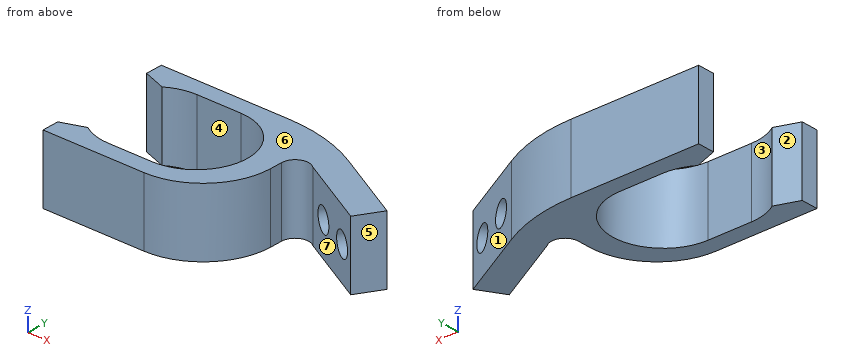
from build123d import *

# Parameters (mm, degrees)
F1_DEPTH = 5
F2_R     = 1.75
F3_DEPTH = 9.9
F4_R     = 24


# Not quite as in the source:
# - a feature names something its author has since deleted; it is built from what else it names


with BuildPart() as f1:
    # F0 (on Top) → F1 (new body, symmetric)
    with BuildSketch(Plane.XY):
        with BuildLine():
            Line((16.2096246684, 11.2512872423), (0, 20))
            Line((0, 20), (-25, 20))
            Line((-25, 20), (-25, 17.5))
            Line((-25, 17.5), (-17.5, 17.5))
            Line((-17.5, 17.5), (-11, 17.5))
            Line((-11, 17.5), (-3.5, 17.5))
            Line((-3.5, 17.5), (-3.5, 10))
            Line((-3.5, 10), (-3.5, 2.5))
            Line((-3.5, 2.5), (-11, 2.5))
            Line((-11, 2.5), (-17.5, 2.5))
            Line((-17.5, 2.5), (-25, 2.5))
            Line((-25, 2.5), (-25, 0))
            Line((-25, 0), (-10, 0))
            ThreePointArc((-10, 0), (-2.9289321881, 2.9289321881), (0, 10))
            Line((0, 10), (0, 11.8892861952))
            ThreePointArc((0, 11.8892861952), (1.1623016269, 13.7053978206), (3.2982614357, 13.4106399491))
            Line((3.2982614357, 13.4106399491), (14.0066361954, 7.6310801635))
            Line((14.0066361954, 7.6310801635), (16.2096246684, 11.2512872423))
        make_face()
        with BuildLine():
            Line((-17.5, 17.5), (-25, 17.5))
            Line((-25, 17.5), (-21.614659653, 16.270532349))
            ThreePointArc((-21.614659653, 16.270532349), (-19.6472083483, 17.186062643), (-17.5, 17.5))
        make_face()
        with BuildLine():
            Line((-21.614659653, 3.729467651), (-25, 2.5))
            Line((-25, 2.5), (-17.5, 2.5))
            ThreePointArc((-17.5, 2.5), (-19.6472083483, 2.813937357), (-21.614659653, 3.729467651))
        make_face()
        with BuildLine():
            Line((-3.5, 17.5), (-11, 17.5))
            ThreePointArc((-11, 17.5), (-5.6966991411, 15.3033008589), (-3.5, 10))
            Line((-3.5, 10), (-3.5, 17.5))
        make_face()
        with BuildLine():
            Line((-3.5, 2.5), (-3.5, 10))
            ThreePointArc((-3.5, 10), (-5.6966991411, 4.6966991411), (-11, 2.5))
            Line((-11, 2.5), (-3.5, 2.5))
        make_face()
    extrude(amount=F1_DEPTH, both=True)

    # F2 (on face) → F3 (cut)
    with BuildSketch(Plane(origin=(8.3593712251, 15.4882522465, 0), x_dir=(-0.8800071661, 0.4749604064, 0), z_dir=(0.4749604064, 0.8800071661, 0))):
        with Locations((-5.9206699059, 0)):
            Circle(F2_R)
        with Locations((0.0793300941, 0)):
            Circle(F2_R)
    extrude(amount=-F3_DEPTH, mode=Mode.SUBTRACT)

    # F4
    f4_edges = [f1.edges().sort_by_distance(p)[0] for p in [
        (0, 20, 0),
    ]]
    fillet(f4_edges, radius=F4_R)


solid = f1.part
Read the model definition and answer for the solid it produces. Units are mm, in the model's axes. Face numbers are marked on the shaded views. A direction names the side the tool comes from. Round coordinates to 2 decimals unless told otherwise and drop trailing zeros. Write each loop counter-clockwise with the first axis right and the second up, starting at its lowest first coordinate (ties: lowest second). Pieces come first, ordered by that corner, then holes. Notation, with made-up numbers: (41, 28) - (53, 28) arc R20 ccw to (53, 34) - close; hole circle Ø7 at (68.25, 37.5). An arc over 180 degrees is marked (long way). Use a Markdown table: item, result.
(1) The part is cut by section A-A (x = -15.5). Write down the section's boundary in (y, z).
Reported:
| item | result |
|---|---|
| outline | (0, -5) - (2.5, -5) - (2.5, 5) - (0, 5) - close; (17.5, -5) - (20, -5) - (20, 5) - (17.5, 5) - close |
(2) Straight lines are drawn through the part: line 1 along Y through (x, z) = (-14, -1.5); line 2 along X through (y, z) = (11.75, 3.25); line 3 along X through (y, z) = (9, -0.75). For each, find the intervals that lie inside material, in ascending order. Write a range as [from, to].
Reported:
| item | result |
|---|---|
| line 1 | [0, 2.5], [17.5, 20] |
| line 2 | [-3.71, 0], [6.38, 15.29] |
| line 3 | [-3.57, -0.05], [13.38, 14.84] |
(3) The part is cut by section D-D (y = 7). Write down the section's boundary in (x, z).
Reported:
| item | result |
|---|---|
| outline | (-4.13, -5) - (-0.46, -5) - (-0.46, 5) - (-4.13, 5) - close |
(4) The part is cut by section B-B (z = 3.75). Write down the section's boundary in (x, y).
Reported:
| item | result |
|---|---|
| outline | (-25, 0) - (-10, 0) arc R10 ccw to (0, 10) - (0, 11.89) arc R2 cw to (3.3, 13.41) - (14.01, 7.63) - (16.21, 11.25) - (5.34, 17.12) arc R24 ccw to (-6.06, 20) - (-25, 20) - (-25, 17.5) - (-21.61, 16.27) arc R7.5 cw to (-17.5, 17.5) - (-11, 17.5) arc R7.5 cw to (-11, 2.5) - (-17.5, 2.5) arc R7.5 cw to (-21.61, 3.73) - (-25, 2.5) - close |
(5) Each of these flat-tipped pins is pushed along its axis until it touches: pin 1 Ø1 at (x, z) = (-1.5, 1.5) entering from +Y; pin 2 Ø5 at (y, z) = (4.5, -1) entering from +X; pin 3 Ø2 at (y, z) = (11, -0.5) entering from +X. Where does it stop, or does it pass through?
Reported:
| item | result |
|---|---|
| pin 1 | y = 19.65 |
| pin 2 | x = -0.46 |
| pin 3 | x = 16.21 |
(6) The mould has two halves that part along X. Classify the marked faces 4, 5, 6 and 7: released by +X, released by -X, zero draft, split by the parting line, or undercut.
Reported:
| item | result |
|---|---|
| face 4 | undercut |
| face 5 | released by +X |
| face 6 | zero draft |
| face 7 | undercut |
(7) The part is cut by section C-C (x = -20). Write down the section's boundary in (y, z), then the cut area to 3 significant figures.
Reported:
| item | result |
|---|---|
| outline | (0, -5) - (2.93, -5) - (2.93, 5) - (0, 5) - close; (17.07, -5) - (20, -5) - (20, 5) - (17.07, 5) - close |
| area | 58.6 mm2 |
(8) Which of the six approach directions +Z, -Z, +X, -X, +Y, -Y give full straight-line access (tool end or side, diameter ignored) to the marked faces 1, 2 and 3?
Reported:
| item | result |
|---|---|
| face 1 | +Z, -Z, +X, +Y |
| face 2 | +Z, -Z, -X |
| face 3 | +Z, -Z |
